```python
from build123d import *

# Parameters (mm, degrees)
SKETCH3_W           = 170.18
SKETCH3_H           = 95.25
BOSS_EXTRUDE1_DEPTH = 7.62
SKETCH4_W           = 6.35
SKETCH4_H           = 6.35
BOSS_EXTRUDE3_DEPTH = 7.62
SKETCH6_R           = 1.0922
CUT_EXTRUDE1_DEPTH  = 10.16


with BuildPart() as part:
    # Sketch3 → Boss-Extrude1 (new body)
    with BuildSketch(Plane(origin=(0, 0, 0), x_dir=(1, 0, 0), z_dir=(0, 1, 0))):
        Rectangle(SKETCH3_W, SKETCH3_H)
    extrude(amount=BOSS_EXTRUDE1_DEPTH)

    # Sketch4 → Boss-Extrude3 (add)
    with BuildSketch(Plane(origin=(0, 7.62, 0), x_dir=(1, 0, 0), z_dir=(0, 1, 0))):
        with Locations((-85.09, 47.625)):
            Rectangle(SKETCH4_W, SKETCH4_H)
        with Locations((-85.09, -47.625)):
            Rectangle(SKETCH4_W, SKETCH4_H)
        with Locations((85.09, 47.625)):
            Rectangle(SKETCH4_W, SKETCH4_H)
        with Locations((85.09, -47.625)):
            Rectangle(SKETCH4_W, SKETCH4_H)
    extrude(amount=-BOSS_EXTRUDE3_DEPTH)

    # Sketch6 → Cut-Extrude1 (cut)
    with BuildSketch(Plane(origin=(0, 7.62, 0), x_dir=(1, 0, 0), z_dir=(0, 1, 0))):
        with Locations(Location((-85.09, 47.625, 0), (0, 0, 270))):
            Circle(SKETCH6_R)
        with Locations(Location((-85.09, -47.625, 0), (0, 0, 270))):
            Circle(SKETCH6_R)
        with Locations(Location((85.09, -47.625, 0), (0, 0, 270))):
            Circle(SKETCH6_R)
        with Locations(Location((85.09, 47.625, 0), (0, 0, 270))):
            Circle(SKETCH6_R)
    extrude(amount=-CUT_EXTRUDE1_DEPTH, mode=Mode.SUBTRACT)


solid = part.part
```
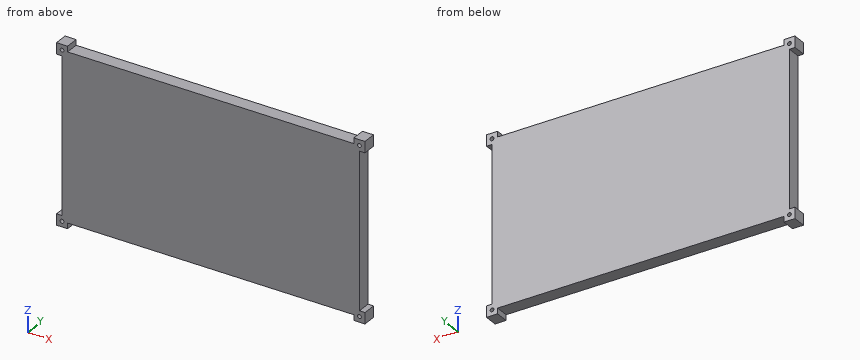
Can you work these out from the model? Positions are in its coordinate system, mm. Give positions to 0.01 mm unless a question says otherwise; leave off trailing zeros. Write each loop counter-clockwise with the first axis right and the second up, starting at its lowest first coordinate (ties: lowest second). Pieces come first, ordered by that corner, then holes. Notation, with made-up numbers: (50, -21) -> (91, -21) arc R17 ccw to (91, 4) -> close; hole circle Ø11 at (55, 57). An arc over 180 degrees is marked (long way). One line per item, written item: value.
Q1. For P1, Ø1.5, axis at x = -17.5, y = 2, coming from the +Z side (3 decimals); P2, Ø1, axis at y = 6, z = -24.5, coming from the -X side; P3, Ø2.5, axis at x = -35.5, y = 5.5, coming from the -Z side (3 decimals), each with a flat end and sliding along its axis, tell me the tip position at first contact or that it passes through.
Results found:
P1: stops at z = 47.625
P2: stops at x = -85.09
P3: stops at z = -47.625
Q2. Please list where these lines run through material, in increasing order: line 1 (X direction, y = 1.5, z = -27.5); line 2 (Z direction, x = -21, y = 2) (3 decimals). Write a range as [from, to].
Results found:
line 1: x = [-85.09, 85.09]
line 2: z = [-47.625, 47.625]
Q3. Imagine slicing it at B-B on z = 11. Please give me the cut outline in (x, y).
Results found:
outline: (-85.09, 0) -> (85.09, 0) -> (85.09, 7.62) -> (-85.09, 7.62) -> close
Q4. Imagine slicing it at A-A on x = -72.5. Please give me the cut outline in (y, z) (3 decimals), and give its area (3 significant figures).
Results found:
outline: (0, -47.625) -> (7.62, -47.625) -> (7.62, 47.625) -> (0, 47.625) -> close
area: 726 mm^2
